Source: three-view drawing plus pictorial views. Frame: mm from the lowest corner of the part. Round coordinates to 2 decimals unless told otherwise and drop trailing zeros. Loops run counter-clockwise (first coordinate to the right, second up) from the corner with the lowest first, then second, coordinate; pieces in that order, holes last. Notation, with made-up numbers: (86.25, 2) -> (142.25, 2) arc R26 cw to (142.25, 41) -> close; hole circle Ø10 at (-1.5, 45.25). An arc over 180 degrees is marked (long way). Answer in a Markdown table with one row per item.
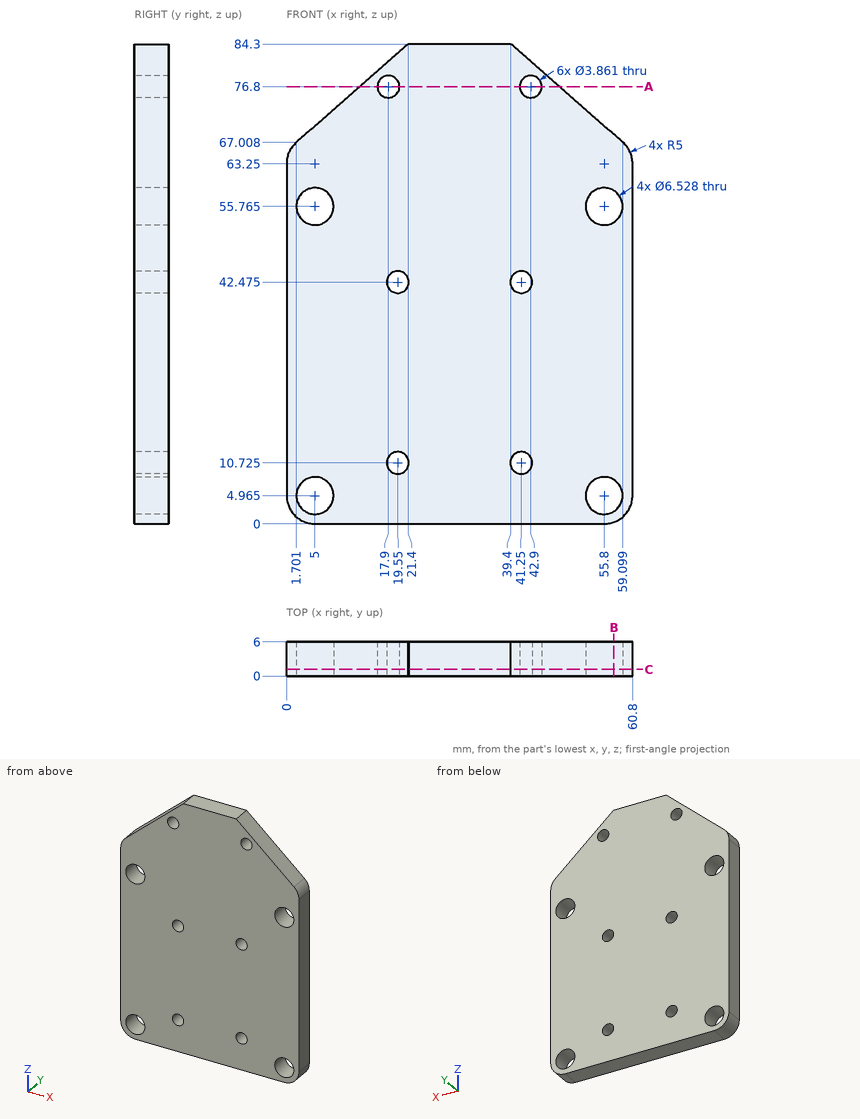
Item 1: Cut plane B-B (x = 57.5). Output: boundary loops of the cut face in (y, z).
Answer:
| item | result |
|---|---|
| outline | (0, 0.3) -> (6, 0.3) -> (6, 2.18) -> (0, 2.18) -> close; (0, 7.75) -> (6, 7.75) -> (6, 52.98) -> (0, 52.98) -> close; (0, 58.55) -> (6, 58.55) -> (6, 68.41) -> (0, 68.41) -> close |
Item 2: Cut plane C-C (y = 1.15). Count the separate pieces of the cut face and the enclosed holes in it, then the cut area to 3 significant figures.
Answer:
| item | result |
|---|---|
| separate pieces | 1 |
| enclosed holes | 10 |
| area | 4,510 mm² |
Item 3: Line query: probe 1 along Z at (x, y) = (19.55, 1.6) (1 decimal); probe 2 along Z at (x, y) = (5, 1.5) (1 decimal); probe 3 along X at (y, z) = (2.4, 76.5) (1 decimal). Output: solid intervals per line, ascending. Write a range as [from, to].
Answer:
| item | result |
|---|---|
| probe 1 | z = [0, 8.8], [12.7, 40.5], [44.4, 75.8], [77.8, 82.7] |
| probe 2 | z = [0, 1.7], [8.2, 52.5], [59, 69.9] |
| probe 3 | x = [12.5, 16], [19.8, 41], [44.8, 48.3] |
Item 4: Cut plane A-A (z = 76.8). Output: boundary loops of the cut face in (x, y), then the cut area to 3 significant figures.
Answer:
| item | result |
|---|---|
| outline | (12.86, 0) -> (15.97, 0) -> (15.97, 6) -> (12.86, 6) -> close; (19.83, 0) -> (40.97, 0) -> (40.97, 6) -> (19.83, 6) -> close; (44.83, 0) -> (47.94, 0) -> (47.94, 6) -> (44.83, 6) -> close |
| area | 164 mm² |
